The drawing under review shows one solid part. Ordinate dimensions are in mm from its lowest x, y, z. A direction names the side the tool comes from. Give positions to 0.01 mm unless a question says otherwise; leave off trailing zeros. Order: outer loops, then holes, each group sorted by start corner. A loop starts at its lowest first (then second) coordinate and runs counter-clockwise, first axis right, second up. Notation, with made-up numbers: (87.5, -3.5) - (113.5, -3.5) arc R21 ccw to (113.5, 10.5) - close; hole circle Ø3 at (71.25, 71). An arc over 180 degrees is marked (long way). Use CSV: the item, a comma, the result in double quotes.
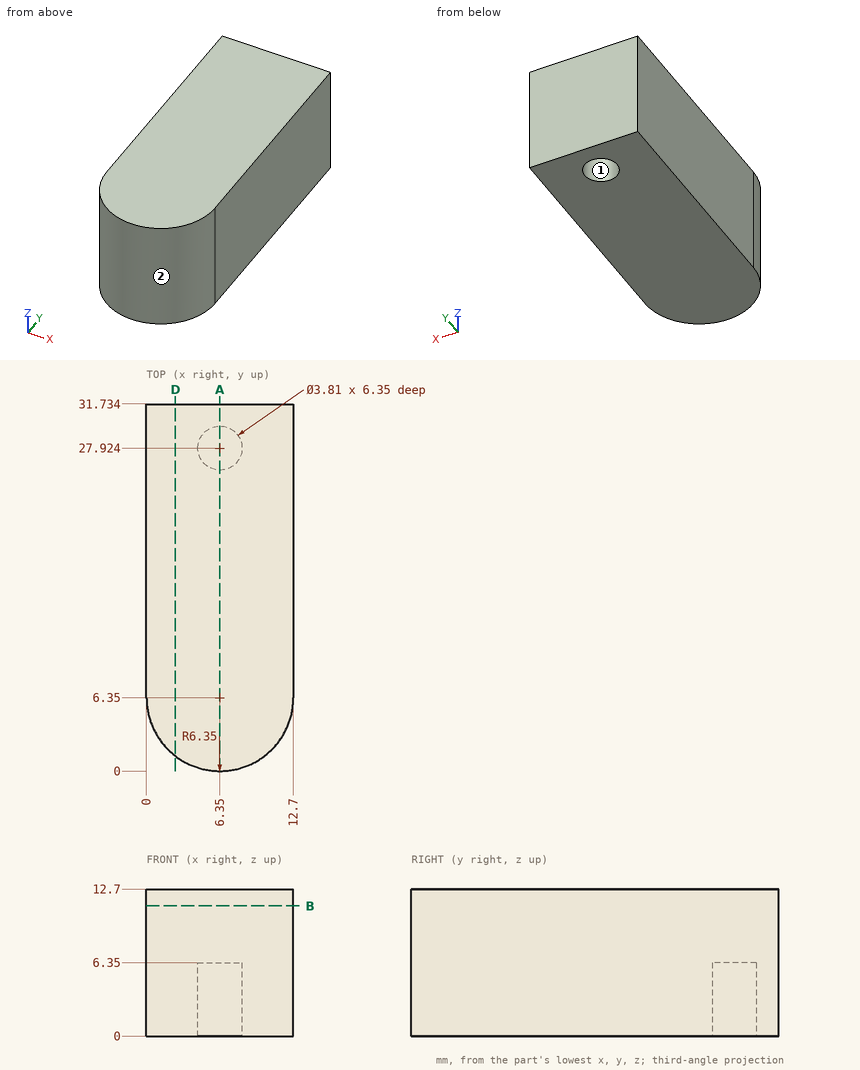
Item 1: Take a section at D-D, the plane x = 2.5. Give the boundary of the cut face in (y, z), and give its area (4 significant figures).
Results list:
outline,"(1.3, 0) - (31.73, 0) - (31.73, 12.7) - (1.3, 12.7) - close"
area,"386.5 mm2"
Item 2: Take a section at A-A, the plane x = 6.35. Give the boundary of the cut face in (y, z).
Results list:
outline,"(0, 0) - (26.02, 0) - (26.02, 6.35) - (29.83, 6.35) - (29.83, 0) - (31.73, 0) - (31.73, 12.7) - (0, 12.7) - close"
Item 3: Wall thickness on L1, parallel to Y at x = 6.35, z = 2.5; L2, parallel to X at y = 28, z = 3.25; L3, parallel to Z at x = 6.5, y = 28: over which ranges is each line inside the solid? List them lowest first.
Results list:
L1,"y = 0 to 26.02, 29.83 to 31.73"
L2,"x = 0 to 4.45, 8.25 to 12.7"
L3,"z = 6.35 to 12.7"
Item 4: Tool access review of the marked faces 1 and 2: name each direction out of +Z, -Z, +X, -X, +Y, -Y from which nothing blocks a thin tool from reaching the whole face with its end or side.
Results list:
face 1,"-Z"
face 2,"+Z, -Z, -Y"
Item 5: Take a section at B-B, the plane z = 11.25. Give the boundary of the cut face in (x, y), and give its area (3 significant figures).
Results list:
outline,"(0, 6.33) arc R6.35 ccw to (12.7, 6.33) - (12.7, 31.73) - (0, 31.73) - close"
area,"386 mm2"
